Can you work these out from the drawing? Everything is in mm from the part's minimum corner. Coordinates: 2 decimals unless noted, no trailing zeros. Loops run counter-clockwise (first coordinate to the right, second up) from the corner with the lowest first, then second, coordinate; pieces in that order, holes last.
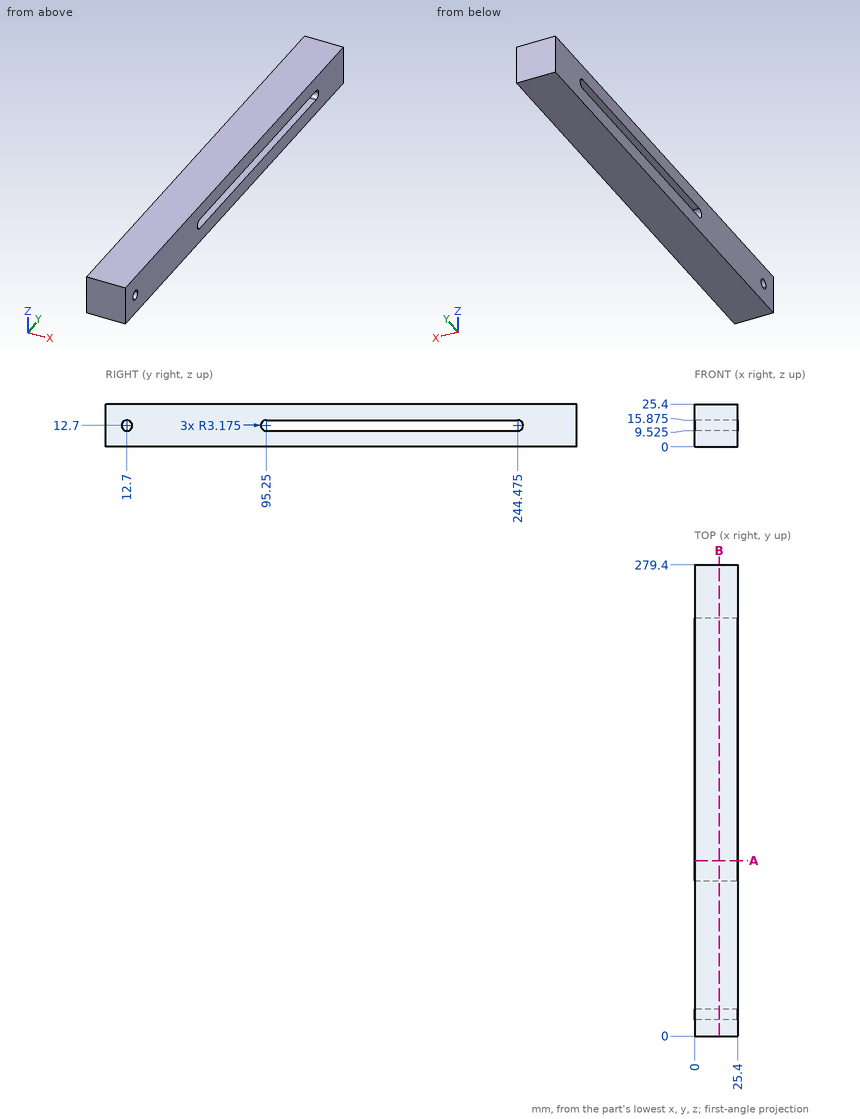
(1) I need wall thicknesses on probe 1 along Y at (x, z) = (23, 12.5); probe 2 along Z at (x, y) = (7.5, 132.5) (3 decimals); probe 3 along Y at (x, z) = (9.75, 11). Which ranges of each line are inside material? Lowest first, please.
Answers:
probe 1: y = 0 to 9.53, 15.87 to 92.08, 247.64 to 279.4
probe 2: z = 0 to 9.525, 15.875 to 25.4
probe 3: y = 0 to 10.02, 15.38 to 92.57, 247.16 to 279.4
(2) Imagine slicing it at A-A, the plane y = 104. Write out the boundary of the cut face in (x, z) (3 decimals).
Answers:
outline: (0, 0) - (25.4, 0) - (25.4, 9.525) - (0, 9.525) - close; (0, 15.875) - (25.4, 15.875) - (25.4, 25.4) - (0, 25.4) - close
(3) Imagine slicing it at B-B, the plane x = 14.5. Write out the boundary of the cut face in (y, z) (3 decimals).
Answers:
outline: (0, 0) - (279.4, 0) - (279.4, 25.4) - (0, 25.4) - close; hole circle Ø6.35 at (12.7, 12.7); hole (95.25, 9.525) - (244.475, 9.525) arc R3.175 ccw to (244.475, 15.875) - (95.25, 15.875) arc R3.175 ccw to start
